Source: CAD feature listing. Evaluate the final solid. Frame: model axes, mm. Give positions to 0.01 mm unless a question says otherwise; leave off trailing zeros. Loops run counter-clockwise (first coordinate to the right, second up) from the corner with the lowest first, then second, coordinate; pieces in that order, holes last. Notation, with made-up numbers: M 22,19.25 L 78,19.25 A16 cw 78,34.25 Z; hole C 89,76 d6. An arc over 180 degrees is marked long. Answer in a Markdown table with one row per item.
Autodesk Inventor part; units mm, degrees
ref_plane "Arbeitsebene1" through (3.25, 0, 0) normal (1, 0, 0) x (0, 1, 0)
ref_plane "XZ Plane" through (0, 0, 0) normal (0, 1, 0) x (-1, 0, 0)
ref_plane "XY Plane" through (0, 0, 0) normal (0, 0, 1) x (1, 0, 0)
sketch "Skizze1" plane through (0, 0, 0) normal (0, 1, 0) x (-1, 0, 0)
  circle A0 centre (0, 0) radius 3.25
  dimension "d0" = 6.5
extrude "Extrusion1" add sketch "Skizze1" along normal blind 30
chamfer "Fasen1" distance 0.5 angle 45 2 edges at (3.25, 30, 0) (3.25, 0, 0)
ref_plane "Arbeitsebene1" through (3.25, 0, 0) normal (1, 0, 0) x (0, 1, 0)
sketch "Skizze2" plane through (3.25, 0, 0) normal (1, 0, 0) x (0, 1, 0)
  line L0 (0, -2.75) -> (0, 2.75)
  line L1 (30, 2.75) -> (30, -2.75)
  point P0 (0, 0)
  point P1 (26, 0)
  point P2 (0, 0)
  dimension "d8" = 4
hole "Bohrung1" at (3.25, 26, 0) direction (-1, 0, 0) diameter 2.5 end through all
properties part number "BMS_bolts" material "Edelstahl"
Q1. Section query C-C (y = 26). Output: boundary loops of the cut face in (x, z), plus the area to 3 significant figures.
Values follow:
| item | result |
|---|---|
| outline | M -3,-1.25 A3.25 ccw 3,-1.25 Z; M -3,1.25 L 3,1.25 A3.25 ccw Z |
| area | 17.3 mm^2 |
Q2. Ray query, probe 1 along Y at (x, z) = (-1.5, 0); probe 2 along Y at (x, z) = (-2, 1); probe 3 along Z at (x, y) = (-0.25, 26). Return the intervals inside material, ascending. Write a range as from..to.
Values follow:
| item | result |
|---|---|
| probe 1 | 0..24.75, 27.25..30 |
| probe 2 | 0..25.25, 26.75..30 |
| probe 3 | -3.24..-1.25, 1.25..3.24 |
Q3. Mould query, pull axis Z, two halves, no side actions, for faces 1 (the flat face through (0, 30, 0)), 2 (the cylindrical face through (2.579, 14.797, 1.978)), 3 (the cylindrical face through (-0.05, 27.22, 0.27)). Classes: +Z half, -Z half, draft (parallel to the pull), parting line (faces both ways), or undercut.
Values follow:
| item | result |
|---|---|
| face 1 | draft |
| face 2 | parting line |
| face 3 | undercut |
Q4. Section query A-A (z = 0). Output: boundary loops of the cut face in (x, y), plus the area to 3 significant figures.
Values follow:
| item | result |
|---|---|
| outline | M -3.25,0.5 L -2.75,0 L 2.75,0 L 3.25,0.5 L 3.25,24.75 L -3.25,24.75 Z; M -3.25,27.25 L 3.25,27.25 L 3.25,29.5 L 2.75,30 L -2.75,30 L -3.25,29.5 Z |
| area | 178 mm^2 |
Q5. Section query B-B (x = 0). Output: boundary loops of the cut face in (y, z), plus the area to 3 significant figures.
Values follow:
| item | result |
|---|---|
| outline | M 0,-2.75 L 0.5,-3.25 L 29.5,-3.25 L 30,-2.75 L 30,2.75 L 29.5,3.25 L 0.5,3.25 L 0,2.75 Z; hole C 26,0 d2.5 |
| area | 190 mm^2 |
Q6. Contact query for a flat-ended pin moving along its axis: pin 1 Ø1.5 at (y, z) = (12, -1.5) entering from -X. Output: stop coordinate, or through.
Values follow:
| item | result |
|---|---|
| pin 1 | x = -3.16 |
